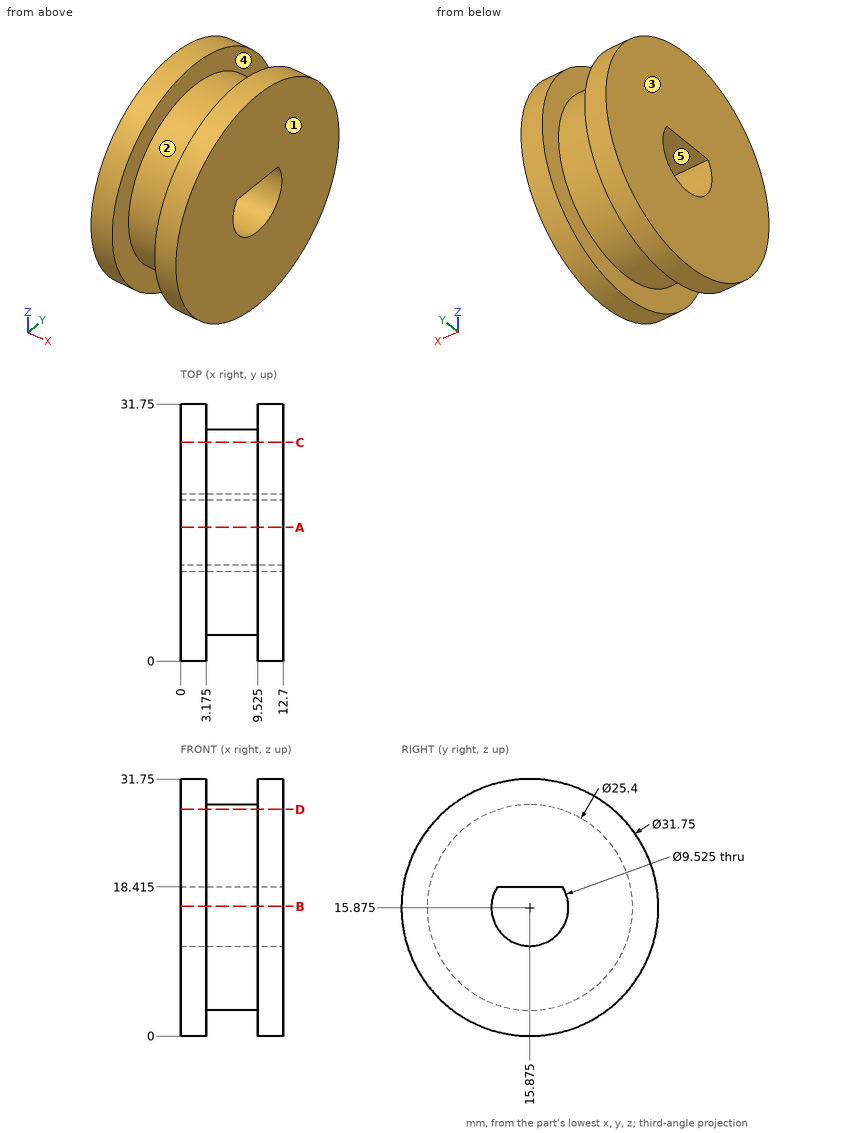
Print and shaded views of the part. All mm, measured from the part's lowest x, y and z. A direction names the side the tool comes from. Give positions to 0.01 mm unless a question says otherwise; leave off trailing zeros. Loops run counter-clockwise (first coordinate to the right, second up) from the corner with the lowest first, then second, coordinate; pieces in that order, holes last. Notation, with made-up numbers: (-38, -28.5) - (2, -28.5) arc R25 cw to (2, -2.5) - close; hole circle Ø2 at (-31, 89). An arc over 180 degrees is marked (long way). Use a Markdown table: item, result.
(1) Band-saw the part on A-A (y = 16.5). Give the cut face in (x, z) (3 decimals).
Taken from the geometry:
| item | result |
|---|---|
| outline | (0, 0.012) - (3.175, 0.012) - (3.175, 3.19) - (9.525, 3.19) - (9.525, 0.012) - (12.7, 0.012) - (12.7, 11.154) - (0, 11.154) - close; (0, 18.415) - (12.7, 18.415) - (12.7, 31.738) - (9.525, 31.738) - (9.525, 28.56) - (3.175, 28.56) - (3.175, 31.738) - (0, 31.738) - close |
(2) Which spindle directions (+Z, -Z, +X, -X, +Y, -Y) get a long thin tool onto all of the face, cutting with end or side? Do the marked faces 1 and 2. Say none if no direction does.
Taken from the geometry:
| item | result |
|---|---|
| face 1 | +Z, -Z, +X, +Y, -Y |
| face 2 | none |
(3) Drop flat-ended pins along their axis: pin 1 Ø2.5 at (x, y) = (5, 14.5) entering from -Z; pin 2 Ø1 at (x, y) = (8.5, 5.5) entering from -Z; pin 3 Ø4 at (x, z) = (11, 22) entering from +Y. Give the stop position or say it passes through.
Taken from the geometry:
| item | result |
|---|---|
| pin 1 | z = 3.18 |
| pin 2 | z = 7.89 |
| pin 3 | y = 31.2 |
(4) Wall check: line 1 along X through (y, z) = (24, 3) (3 decimals); line 2 along Y through (x, z) = (6, 16.5); line 3 along Y through (x, z) = (5.5, 12). Give the ranges that are in metal, low to high.
Taken from the geometry:
| item | result |
|---|---|
| line 1 | 0 to 3.175, 9.525 to 12.7 |
| line 2 | 3.19 to 11.15, 20.6 to 28.56 |
| line 3 | 3.78 to 13.11, 18.64 to 27.97 |
(5) Band-saw the part on B-B (z = 16). Give the cut face in (x, y) (1 decimal), and give its area (3 significant figures).
Taken from the geometry:
| item | result |
|---|---|
| outline | (0, 0) - (3.2, 0) - (3.2, 3.2) - (9.5, 3.2) - (9.5, 0) - (12.7, 0) - (12.7, 11.1) - (0, 11.1) - close; (0, 20.6) - (12.7, 20.6) - (12.7, 31.7) - (9.5, 31.7) - (9.5, 28.6) - (3.2, 28.6) - (3.2, 31.7) - (0, 31.7) - close |
| area | 242 mm2 |
(6) Band-saw the part on C-C (y = 27). Give the cut face in (x, z) (3 decimals).
Taken from the geometry:
| item | result |
|---|---|
| outline | (0, 4.55) - (3.175, 4.55) - (3.175, 9.749) - (9.525, 9.749) - (9.525, 4.55) - (12.7, 4.55) - (12.7, 27.2) - (9.525, 27.2) - (9.525, 22.001) - (3.175, 22.001) - (3.175, 27.2) - (0, 27.2) - close |
(7) Pull direction X, two halves, no side cores. Call the marked faces 3, 4 and 5: +X half, -X half, draft (parallel to the pull), parting line (faces both ways), or undercut.
Taken from the geometry:
| item | result |
|---|---|
| face 3 | -X half |
| face 4 | undercut |
| face 5 | draft |
(8) Band-saw the part on D-D (z = 28). Give the cut face in (x, y) (3 decimals), and give its area (3 significant figures).
Taken from the geometry:
| item | result |
|---|---|
| outline | (0, 5.628) - (3.175, 5.628) - (3.175, 12.097) - (9.525, 12.097) - (9.525, 5.628) - (12.7, 5.628) - (12.7, 26.122) - (9.525, 26.122) - (9.525, 19.653) - (3.175, 19.653) - (3.175, 26.122) - (0, 26.122) - close |
| area | 178 mm2 |
